```python
from build123d import *

# Parameters (mm, degrees)
F10_DEPTH = 2
F11_DEPTH = 2
F12_DEPTH = 2
F13_DEPTH = 2
F14_W     = 8.485019207
F14_H     = 5.5162683129
F15_DEPTH = 25.4
F16_W     = 22.2342889756
F16_H     = 4.6487008221
F17_DEPTH = 25.4
F18_W     = 7.9449899495
F18_H     = 7.2886322159
F19_DEPTH = 25.4
F20_W     = 5.9225577861
F20_H     = 11.3939000294
F21_DEPTH = 25.4
F22_DEPTH = 25.4
F24_DEPTH = 2
F25_W     = 2.8602282982
F25_H     = 1.0062001161
F26_DEPTH = 25.4


with BuildPart() as f10:
    # F9 (on 3pt) → F10 (new body)
    with BuildSketch(Plane(origin=(3.3858576339, 10.4205982991, 0.8801059814), x_dir=(-0.9513782964, 0.3069321376, 0.0259229655), z_dir=(0.308024897, 0.9480031547, 0.0800667316))):
        Polygon((7.9863190401, -1.0910055423), (-27.9953896476, 21.7198480533), (-8.0322433603, -0.6742785071), align=None)
    extrude(amount=-F10_DEPTH)

    # F7 (on 3pt) → F11 (join)
    with BuildSketch(Plane(origin=(-2.4612159584, 1.7881780643, 4.9288143129), x_dir=(0.9052277817, 0.144920932, 0.3994503557), z_dir=(-0.4249266563, 0.3087272871, 0.8509552274))):
        Polygon((35.8818855958, -7.4339114282), (-1.9342501918, 12.1864421859), (-12.3389909213, 0), align=None)
    extrude(amount=-F11_DEPTH)

    # F6 (on 3pt) → F12 (join)
    with BuildSketch(Plane(origin=(-2.4612159584, -1.7881780643, 4.9288143129), x_dir=(0.9052277817, -0.144920932, 0.3994503557), z_dir=(-0.4249266563, -0.3087272871, 0.8509552274))):
        Polygon((-1.9342501918, -12.1864421859), (35.8818855958, 7.4339114282), (-12.3389909213, 0), align=None)
    extrude(amount=-F12_DEPTH)

    # F5 (on face) → F13 (join)
    with BuildSketch(Plane(origin=(3.3858576339, -10.4205982991, 0.8801059814), x_dir=(0.9513782964, 0.3069321376, -0.0259229655), z_dir=(0.308024897, -0.9480031547, 0.0800667316))):
        Polygon((8.0322433603, -0.6742785071), (27.9953896476, 21.7198480533), (-7.9863190401, -1.0910055423), align=None)
    extrude(amount=-F13_DEPTH)

    # F14 (on face) → F15 (cut)
    with BuildSketch(Plane(origin=(3.3858576339, -10.4205982991, 0.8801059814), x_dir=(0.9513782964, 0.3069321376, -0.0259229655), z_dir=(0.308024897, -0.9480031547, 0.0800667316))):
        with Locations((25.7894098759, 19.5572990924)):
            Rectangle(F14_W, F14_H)
    extrude(amount=F15_DEPTH, mode=Mode.SUBTRACT)

    # F16 (on face) → F17 (cut)
    with BuildSketch(Plane(origin=(-2.4612159584, 1.7881780643, 4.9288143129), x_dir=(0.9052277817, 0.144920932, 0.3994503557), z_dir=(-0.4249266563, 0.3087272871, 0.8509552274))):
        with Locations((32.4524613097, -6.6612462979)):
            Rectangle(F16_W, F16_H)
    extrude(amount=F17_DEPTH, mode=Mode.SUBTRACT)

    # F18 (on face) → F19 (cut)
    with BuildSketch(Plane(origin=(-2.4612159584, -1.7881780643, 4.9288143129), x_dir=(0.9052277817, -0.144920932, 0.3994503557), z_dir=(-0.4249266563, -0.3087272871, 0.8509552274))):
        with Locations((35.5167929083, 5.7378442725)):
            Rectangle(F18_W, F18_H)
    extrude(amount=F19_DEPTH, mode=Mode.SUBTRACT)

    # F20 (on face) → F21 (cut)
    with BuildSketch(Plane(origin=(3.3858576339, 10.4205982991, 0.8801059814), x_dir=(-0.9513782964, 0.3069321376, 0.0259229655), z_dir=(0.308024897, 0.9480031547, 0.0800667316))):
        with Locations((-26.7476057634, 18.5779468156)):
            Rectangle(F20_W, F20_H)
    extrude(amount=F21_DEPTH, mode=Mode.SUBTRACT)

    # F0 (on Top) → F22 (cut)
    with BuildSketch(Plane.XY):
        Polygon((11.027559638, -8.0119910571), (11.027559638, 8.0119910571), (-4.2121529688, 12.963673848), (-13.6308133385, 0), (-4.2121529688, -12.963673848), align=None)
    extrude(amount=-F22_DEPTH, mode=Mode.SUBTRACT)

    # F23 (on face) → F24 (join)
    with BuildSketch(Plane(origin=(0, 0, 0), x_dir=(1, 0, 0), z_dir=(0, 0, -1))):
        Polygon((6.725183616, 3.5935375892), (6.725183616, -3.5935375892), (10.5510387165, -6.0571244693), (10.5510387165, 6.0571244693), align=None)
        Polygon((10.5510387165, -6.0571244693), (6.725183616, -3.5935375892), (6.725183616, -7.3002201464), align=None)
        Polygon((6.725183616, 7.3002201464), (6.725183616, 3.5935375892), (10.5510387165, 6.0571244693), align=None)
    extrude(amount=-F24_DEPTH)

    # F25 (on face) → F26 (cut)
    with BuildSketch(Plane(origin=(6.725183616, 0, 0), x_dir=(0, -1, 0), z_dir=(-1, 0, 0))):
        Polygon((2.8602282982, 2), (2.8602282982, 0.9937998839), (4.1250204667, 2), align=None)
        with Locations((1.4301141491, 1.4968999419)):
            Rectangle(F25_W, F25_H)
        with Locations((-1.4301141491, 1.4968999419)):
            Rectangle(F25_W, F25_H)
        Polygon((-4.1250204667, 2), (-2.8602282982, 0.9937998839), (-2.8602282982, 2), align=None)
    extrude(amount=-F26_DEPTH, mode=Mode.SUBTRACT)


solid = f10.part
```
Part model, mm, in its own coordinate system. A direction names the side the tool comes from. Round coordinates to 2 decimals unless told otherwise and drop trailing zeros. Loops run counter-clockwise (first coordinate to the right, second up) from the corner with the lowest first, then second, coordinate; pieces in that order, holes last. Notation, with made-up numbers: (49, 21) -> (85, 21) arc R22 cw to (85, 27) -> close; hole circle Ø5 at (-5.5, 66.25). An arc over 180 degrees is marked (long way). Use CSV: the item, a comma, the result in double quotes. Start each with the question number.
1) Which spindle directions (+Z, -Z, +X, -X, +Y, -Y) get a long thin tool onto all of the face, cutting with end or side? Do faces 1 (the flat face through (28.82, 0.42, 19.75)), 2 (the flat face through (9, 0, 0.994)), 3 (the flat face through (5.37, 3.52, 5.86)), 4 (the flat face through (26.856, -0.643, 17.634)), 5 (the flat face through (28.81, -0.42, 19.74)). Say none if no direction does.
2) Cut at D-D, the plane x = -2.5. Write the cut outline in (y, z), plus the area to 3 significant figures.
3) Drop flat-ended pins along their axis: P1, Ø6, axis at x = -6, y = 3, coming from the +Z side; P2, Ø1.5, axis at y = 4, z = 9, coming from the +X side; P3, Ø1, axis at x = 17, y = -5.5, coming from the -Z side. Give the stop position or say it passes through.
4) Wall check: L1, parallel to Y at x = 10, z = 4; L2, parallel to Z at x = 8, y = 4.25; L3, parallel to X at y = 3.25, z = 11.75. Give the ranges that are in metal, low to high. Write a range as [from, to].
5) Cut at B-B, the plane x = 8. Write the cut outline in (y, z), plus the area to 3 significant figures.
6) Cut at C-C, the plane z = 4. Write the cut outline in (x, y).
7) Pull direction Y, two halves, no side cores. Call faces 6 (the flat face through (17.98, -4.02, 8.25)), 7 (the flat face through (12.98, 6.81, 6.74)), 8 (the flat face through (28.8, -0.34, 18.96)): +Y half, -Y half, draft (parallel to the pull), parting line (faces both ways), or undercut.
8) Cut at A-A, the plane y = 4.75. Write the cut outline in (x, z), plus the area to 3 significant figures.
Determined:
1,face 1,"+Y"
1,face 2,"+X"
1,face 3,"none"
1,face 4,"-Z, +X"
1,face 5,"-Y"
2,outline,"(-12.41, 0) -> (-8.84, 0) -> (0, 3.21) -> (8.84, 0) -> (12.41, 0) -> (12.32, 1.09) -> (0, 5.56) -> (-12.32, 1.09) -> close"
2,area,"53.6 mm2"
3,P1,"stops at z = 4.57"
3,P2,"stops at x = 19.44"
3,P3,"stops at z = 6.32"
4,L1,"y = [-8.01, -5.9], [5.9, 8.01]"
4,L2,"z = [0, 2], [6.91, 9.26]"
4,L3,"x = [12.26, 21.16]"
5,outline,"(-9, 0) -> (9, 0) -> (8.34, 7.78) -> (0, 10.8) -> (-8.34, 7.78) -> close; hole (-6.72, 2) -> (-4.13, 2) -> (-2.86, 0.99) -> (2.86, 0.99) -> (4.13, 2) -> (6.72, 2) -> (6.37, 6.14) -> (0, 8.45) -> (-6.37, 6.14) -> close"
5,area,"84.1 mm2"
6,outline,"(-5.62, 0) -> (2.07, -10.58) -> (14.51, -6.54) -> (14.04, -4.59) -> (4.64, -7.64) -> (-0.91, 0) -> (4.64, 7.64) -> (14.04, 4.59) -> (14.51, 6.54) -> (2.07, 10.58) -> close"
7,face 6,"undercut"
7,face 7,"+Y half"
7,face 8,"-Y half"
8,outline,"(-10.18, 0) -> (-5.47, 0) -> (12.27, 8.86) -> (13.65, 3.56) -> (18.76, 8.87) -> (17.48, 13.81) -> close; (6.73, 0) -> (10.55, 0) -> (10.55, 2) -> (6.73, 2) -> close"
8,area,"94.2 mm2"
